Geometry check sheet. Reference: the model listing, model coordinates, mm. A direction names the side the tool comes from. Give positions to 0.01 mm unless a question says otherwise; leave off trailing zeros. Order: outer loops, then holes, each group sorted by start corner. A loop starts at its lowest first (then second) coordinate and runs counter-clockwise, first axis right, second up. Notation, with made-up numbers: (59.25, 69.25) - (70.25, 69.25) arc R38 ccw to (70.25, 107.25) - close; hole circle Ø11 at (26, 19). An arc over 180 degrees is marked (long way). Put each result on its own line as item: value. Start each with the question number.
```python
from build123d import *
from build123d.topology import SkipClean

# Parameters (mm, degrees)
EXTRUDE_1_OUTLINE_R      = 2.6
EXTRUDE_1_DEPTH          = 8
CUT_EXTRUDE_1_DEPTH      = 50.836100116
CUT_EXTRUDE_1_DEPTH_BACK = 50.836100116
SKETCH_2_R               = 1.4
EXTRUDE_START            = 1
SKETCH_3_R               = 4
SKETCH_3_R_2             = 2.6
EXTRUDE_2_DEPTH          = 1
FILLET_1_R               = 3
CHAMFER_1_SIZE           = 3


# Read off the part's stored shape, not the designer's step: 凸台-拉伸1
with BuildPart() as part:
    # 凸台-拉伸1 outline → 凸台-拉伸1 (new body)
    with BuildSketch(Plane(origin=(0, 0, 0), x_dir=(1, 0, 0), z_dir=(0, 1, 0))):
        with BuildLine():
            ThreePointArc((-27.888081975, 11.234427543), (-26.242200252, 9.598392892), (-24, 9))
            ThreePointArc((-24, 9), (-15.136730223, 1.562833599), (-20.92181871, -8.457233587))
            Line((-20.92181871, -8.457233587), (-33.550042142, -13.053531028))
            ThreePointArc((-33.550042142, -13.053531028), (-32.755177906, -14.936476169), (-31.854736566, -16.771277779))
            ThreePointArc((-31.854736566, -16.771277779), (-27.859752737, -18.097023194), (-23.673340637, -18.534573681))
            ThreePointArc((-23.673340637, -18.534573681), (-21.433552206, -17.927215624), (-19.794228634, -16.284609691))
            ThreePointArc((-19.794228634, -16.284609691), (-8.92181871, -12.327376104), (-3.136730223, -22.34744329))
            Line((-3.136730223, -22.34744329), (-5.470331592, -35.581954307))
            ThreePointArc((-5.470331592, -35.581954307), (-3.442221148, -35.835054257), (-1.403015673, -35.972649986))
            ThreePointArc((-1.403015673, -35.972649986), (1.742605451, -33.17576521), (4.214741338, -29.769001224))
            ThreePointArc((4.214741338, -29.769001224), (4.808648047, -27.525608515), (4.205771366, -25.284609691))
            ThreePointArc((4.205771366, -25.284609691), (6.214911513, -13.890209703), (17.785088487, -13.890209703))
            Line((17.785088487, -13.890209703), (28.07971055, -22.528423279))
            ThreePointArc((28.07971055, -22.528423279), (29.312956758, -20.898578088), (30.451720893, -19.201372207))
            ThreePointArc((30.451720893, -19.201372207), (29.602358188, -15.078742016), (27.888081975, -11.234427543))
            ThreePointArc((27.888081975, -11.234427543), (26.242200252, -9.598392892), (24, -9))
            ThreePointArc((24, -9), (15.136730223, -1.562833599), (20.92181871, 8.457233587))
            Line((20.92181871, 8.457233587), (33.550042142, 13.053531028))
            ThreePointArc((33.550042142, 13.053531028), (32.755177906, 14.936476169), (31.854736566, 16.771277779))
            ThreePointArc((31.854736566, 16.771277779), (27.859752737, 18.097023194), (23.673340637, 18.534573681))
            ThreePointArc((23.673340637, 18.534573681), (21.433552206, 17.927215624), (19.794228634, 16.284609691))
            ThreePointArc((19.794228634, 16.284609691), (8.92181871, 12.327376104), (3.136730223, 22.34744329))
            Line((3.136730223, 22.34744329), (5.470331592, 35.581954307))
            ThreePointArc((5.470331592, 35.581954307), (3.442221148, 35.835054257), (1.403015673, 35.972649986))
            ThreePointArc((1.403015673, 35.972649986), (-1.742605451, 33.17576521), (-4.214741338, 29.769001224))
            ThreePointArc((-4.214741338, 29.769001224), (-4.808648047, 27.525608515), (-4.205771366, 25.284609691))
            ThreePointArc((-4.205771366, 25.284609691), (-6.214911513, 13.890209703), (-17.785088487, 13.890209703))
            Line((-17.785088487, 13.890209703), (-28.07971055, 22.528423279))
            ThreePointArc((-28.07971055, 22.528423279), (-29.312956758, 20.898578088), (-30.451720893, 19.201372207))
            ThreePointArc((-30.451720893, 19.201372207), (-29.602358188, 15.078742016), (-27.888081975, 11.234427543))
        make_face()
        Circle(EXTRUDE_1_OUTLINE_R, mode=Mode.SUBTRACT)
    extrude(amount=EXTRUDE_1_DEPTH)

    # 草图2 → 切除-拉伸1 (cut, two sides: drawn at the far end of the back side and taken through both)
    with BuildSketch(Plane(origin=(0, 0, 0), x_dir=(0, 0, -1), z_dir=(1, 0, 0)).offset(-CUT_EXTRUDE_1_DEPTH_BACK)):
        with Locations((0, 4)):
            Circle(SKETCH_2_R)
    extrude(amount=CUT_EXTRUDE_1_DEPTH + CUT_EXTRUDE_1_DEPTH_BACK, mode=Mode.SUBTRACT)

    # 草图3 → 凸台-拉伸2 (add)
    with SkipClean():  # the faces are left unmerged after this step: merging them gives an invalid solid
        with BuildSketch(Plane.XZ.offset(EXTRUDE_START)):
            with Locations(Location((0, 0, 0), (0, 0, 90))):
                Circle(SKETCH_3_R)
            with Locations(Location((0, 0, 0), (0, 0, 270))):
                Circle(SKETCH_3_R_2, mode=Mode.SUBTRACT)
        extrude(amount=-EXTRUDE_2_DEPTH)

    # 圆角1
    # the kernel refuses this fillet: 3 mm, written as the material it adds along each edge
    with BuildSketch(Plane(origin=(0, 0, 0), x_dir=(0, 0, 1), z_dir=(1, 0, 0))) as fillet_1_piece_1:
        with BuildLine():
            CenterArc((6.236067977, 3), FILLET_1_R, 221.810314896, 48.189685104)
            Line((4, 1), (3.95527864, 0.96))
            ThreePointArc((3.95527864, 0.96), (3.94, 0.5), (3.94, 0))
            Line((3.94, 0), (4, -0.06))
            Line((4, -0.06), (6.236067977, -0.06))
            Line((6.236067977, -0.06), (6.236067977, 0))
        make_face()
    revolve(axis=Axis((0, 0, 0), (0, -1, 0)))

    # 倒角1
    # the kernel refuses this chamfer: 3 mm, written as the material it takes off along each edge
    with BuildSketch(Plane(origin=(-23.751350664, 0, -0.965270296), x_dir=(-0.7340128901584542, 0, 0.6791355366060836), z_dir=(-0.6791355366060836, 0, -0.7340128901584542))) as chamfer_1_piece_1:
        Polygon((19.500000018 - CHAMFER_1_SIZE, 0), (19.500000018, CHAMFER_1_SIZE), (19.500000018, 0), align=None)
    revolve(axis=Axis((-23.751350664, 0, -0.965270296), (0, 1, 0)), revolution_arc=70.122480661, mode=Mode.SUBTRACT)
    with BuildSketch(Plane(origin=(-11.039726758, 0, -21.051908187), x_dir=(-0.9551550721197726, 0, -0.29610604216035863), z_dir=(0.29610604216035863, 0, -0.9551550721197726))) as chamfer_1_piece_2:
        Polygon((19.499999992 - CHAMFER_1_SIZE, 0), (19.499999992, CHAMFER_1_SIZE), (19.499999992, 0), align=None)
    revolve(axis=Axis((-11.039726758, 0, -21.051908187), (0, 1, 0)), revolution_arc=70.122480753, mode=Mode.SUBTRACT)
    with BuildSketch(Plane(origin=(12.711623912, 0, -20.086637915), x_dir=(-0.2211421814618006, 0, -0.9752415780606957), z_dir=(0.9752415780606957, 0, -0.2211421814618006))) as chamfer_1_piece_3:
        Polygon((19.499999996 - CHAMFER_1_SIZE, 0), (19.499999996, CHAMFER_1_SIZE), (19.499999996, 0), align=None)
    revolve(axis=Axis((12.711623912, 0, -20.086637915), (0, 1, 0)), revolution_arc=70.122480742, mode=Mode.SUBTRACT)
    with BuildSketch(Plane(origin=(23.751350664, 0, 0.965270296), x_dir=(0.7340128901584542, 0, -0.6791355366060836), z_dir=(0.6791355366060836, 0, 0.7340128901584542))) as chamfer_1_piece_4:
        Polygon((19.500000018 - CHAMFER_1_SIZE, 0), (19.500000018, CHAMFER_1_SIZE), (19.500000018, 0), align=None)
    revolve(axis=Axis((23.751350664, 0, 0.965270296), (0, 1, 0)), revolution_arc=70.122480661, mode=Mode.SUBTRACT)
    with BuildSketch(Plane(origin=(11.039726758, 0, 21.051908187), x_dir=(0.9551550721197726, 0, 0.29610604216035863), z_dir=(-0.29610604216035863, 0, 0.9551550721197726))) as chamfer_1_piece_5:
        Polygon((19.499999992 - CHAMFER_1_SIZE, 0), (19.499999992, CHAMFER_1_SIZE), (19.499999992, 0), align=None)
    revolve(axis=Axis((11.039726758, 0, 21.051908187), (0, 1, 0)), revolution_arc=70.122480753, mode=Mode.SUBTRACT)
    with BuildSketch(Plane(origin=(-12.711623912, 0, 20.086637915), x_dir=(0.2211421814618006, 0, 0.9752415780606957), z_dir=(-0.9752415780606957, 0, 0.2211421814618006))) as chamfer_1_piece_6:
        Polygon((19.499999996 - CHAMFER_1_SIZE, 0), (19.499999996, CHAMFER_1_SIZE), (19.499999996, 0), align=None)
    revolve(axis=Axis((-12.711623912, 0, 20.086637915), (0, 1, 0)), revolution_arc=70.122480742, mode=Mode.SUBTRACT)


solid = part.part
```
Item 1: Set-up check for faces 1 (the face through (-4.287, 3.944, 28.872)), 2 (the face through (21.462, 5.307, -17.944)), 3 (the face through (4.287, 3.944, -28.872)): record each of +Z, -Z, +X, -X, +Y, -Y from which the full face is reachable in a straight line by a thin tool's end or side.
Item 2: Thickness scan on line 1 along X through (y, z) = (0.75, 0); line 2 along X through (y, z) = (3.5, 16.5); line 3 along Y through (x, z) = (7, -6.5). Record the ranges inside material, lowest first.
Item 3: Cross-section at A-A (z = 0). Enter the section's corners in (x, y), and give its area (3 significant figures).
Item 4: Gauge pin test, flat ends, axial feed: pin 1 Ø3 at (x, y) = (23, 0.5) entering from -Z; pin 2 Ø4 at (y, z) = (5, 9) entering from +X; pin 3 Ø6 at (x, z) = (4, -15) entering from -Y; pin 4 Ø8.5 at (x, z) = (0, 0) entering from +Y. Record the tip position at first contact, or that the pin passes through.
Item 5: Release check for a two-part mould opening along Z. For faces 4 (the face through (29.62, 5.46, 15.13)), 5 (the face through (3.471, 5.072, -35.832)), 6 (the face through (-27.917, 5.465, 18.084)) record: +Z half, -Z half, draft (parallel to the pull), parting line (faces both ways), or undercut.
Item 6: Cross-section at C-C (x = 14). Enter the section's corners in (y, z).
Recorded:
1. face 1: -X, +Y, -Y
1. face 2: -Z, +Y, -Y
1. face 3: +X, +Y, -Y
2. line 1: x = -15 to -2.6, 2.6 to 15
2. line 2: x = -32 to -19.93, -4.09 to 4.09, 20.9 to 30
2. line 3: y = 0 to 8
3. outline: (-15, 0) - (-6.24, 0) arc R3 cw to (-4, -1) - (-2.6, -1) - (-2.6, 2.6) - (-15, 2.6) - close; (-15, 5.4) - (-2.6, 5.4) - (-2.6, 8) - (-15, 8) - close; (2.6, -1) - (4, -1) arc R3 cw to (6.24, 0) - (15, 0) - (15, 2.6) - (2.6, 2.6) - close; (2.6, 5.4) - (15, 5.4) - (15, 8) - (2.6, 8) - close
3. area: 133 mm^2
4. pin 1: stops at z = -17.52
4. pin 2: stops at x = 27.74
4. pin 3: stops at y = 0
4. pin 4: stops at y = 8
5. face 4: undercut
5. face 5: -Z half
5. face 6: +Z half
6. outline: (0, -12.01) - (8, -12.01) - (8, 12.01) - (0, 12.01) - close; hole circle Ø2.8 at (4, 0)
